Source: CAD feature listing. Evaluate the final solid. Frame: model axes, mm. Round coordinates to 2 decimals unless told otherwise and drop trailing zeros. Order: outer loops, then holes, each group sorted by start corner. A loop starts at its lowest first (then second) coordinate and runs counter-clockwise, first axis right, second up. Notation, with made-up numbers: (79.5, 41.25) - (130.5, 41.25) arc R16 ccw to (130.5, 52.25) - close; hole circle Ø7 at (-4, 75.5). An arc over 180 degrees is marked (long way). Return JSON: item names as keys, results as strings. Group by question number.
1) Ray query, line 1 (X direction, y = 1.75, z = -31.75) (3 decimals); line 2 (X direction, y = 0.9, z = -12.7); line 3 (X direction, y = 0.75, z = -30) (3 decimals). Return the intervals inside material, ascending. Write a range as from..to.
2) Section D-D, the plane x = -38.1. Return loops of the section in (y, z).
3) Contact query for a flat-ended pin moving along its axis: P1, Ø4, axis at x = -55.5, z = -68, coming from the -Y side. Output: stop coordinate, or through.
4) Section B-B, the plane z = -57.15. Return loops of the section in (x, y).
5) Section A-A, the plane z = -36.5. Return loops of the section in (x, y) (3 decimals), plus the area to 3 significant figures.
6) Section C-C, the plane x = -63.5. Return loops of the section in (y, z), plus the area to 3 significant figures.
Autodesk Inventor part; units mm, degrees
ref_plane "YZ Plane" through (0, 0, 0) normal (1, 0, 0) x (0, 1, 0)
ref_plane "XZ Plane" through (0, 0, 0) normal (0, 1, 0) x (-1, 0, 0)
ref_plane "XY Plane" through (0, 0, 0) normal (0, 0, 1) x (1, 0, 0)
sketch "Sketch1" plane through (0, 0, 0) normal (0, 1, 0) x (-1, 0, 0)
  line L0 (0, 0) -> (76.2, 0)
  line L1 (76.2, 0) -> (76.2, -76.2)
  line L2 (76.2, -76.2) -> (0, -76.2)
  line L3 (0, -76.2) -> (0, 0)
  dimension "d0" = 76.2
  dimension "d1" = 76.2
extrude "Extrusion1" add sketch "Sketch1" along normal blind 2.3813
sketch "Sketch2" plane through (0, 2.3813, 0) normal (0, 1, 0) x (1, 0, 0)
  line L0 (-83.8553, 12.7) -> (21.3104, 12.7) construction
  line L1 (-76.2, 0) -> (0, 0) construction
  line L2 (-76.2, 76.2) -> (-76.2, 0) construction
  point P0 (-63.5, 12.7)
  point P1 (-38.1, 12.7)
  point P2 (-12.7, 12.7)
  dimension "d4" = 12.7
  dimension "d5" = 12.7
  dimension "d6" = 25.4
  dimension "d39" = 25.4
hole "Hole1" at (-63.5, 2.3813, -12.7) at (-38.1, 2.3813, -12.7) at (-12.7, 2.3813, -12.7) direction (0, -1, 0) diameter 4.4958 end through all
sketch "Sketch3" plane through (0, 2.3813, 0) normal (0, 1, 0) x (1, 0, 0)
  line L0 (-85.7811, 31.75) -> (14.4142, 31.75) construction
  line L1 (-76.2, 0) -> (0, 0) construction
  line L2 (-38.1, 80.8292) -> (-38.1, -11.6218) construction
  line L3 (0, 76.2) -> (-76.2, 76.2) construction
  point P0 (-58.3565, 31.75)
  point P1 (-17.8435, 31.75)
  point P2 (-38.1, 76.2)
  dimension "d14" = 31.75
  dimension "d16" = 40.513
hole "Hole2" at (-58.3565, 2.3813, -31.75) at (-17.8435, 2.3813, -31.75) direction (0, -1, 0) diameter 3.175 end through all
sketch "Sketch4" plane through (0, 2.3813, 0) normal (0, 1, 0) x (1, 0, 0)
  line L0 (-58.3565, 76.2) -> (-17.8435, 76.2)
  line L1 (-17.8435, 76.2) -> (-17.8435, 38.1)
  line L2 (-17.8435, 38.1) -> (-58.3565, 38.1)
  line L3 (-58.3565, 38.1) -> (-58.3565, 76.2)
  line L4 (0, 76.2) -> (-76.2, 76.2)
  line L5 (-38.1, 81.963) -> (-38.1, -24.4331)
  line L6 (-76.2, 0) -> (0, 0)
  line L7 (-53.975, 38.1) -> (-22.225, 38.1)
  line L8 (-22.225, 38.1) -> (-22.225, 25.4)
  line L9 (-22.225, 25.4) -> (-53.975, 25.4)
  line L10 (-53.975, 25.4) -> (-53.975, 38.1)
  point P0 (-38.1, 0)
  dimension "d24" = 38.1
  dimension "d27" = 31.75
  dimension "d28" = 12.7
  dimension "d29" = 40.513
extrude "Extrusion2" cut sketch "Sketch4" against normal blind 2.3813
sketch "Sketch5" plane through (0, 2.3813, 0) normal (0, 1, 0) x (1, 0, 0)
  line L0 (-81.1122, 57.15) -> (21.0892, 57.15) construction
  line L1 (-58.3565, 76.2) -> (-76.2, 76.2) construction
  line L2 (-38.1, 88.2697) -> (-38.1, -12.0157) construction
  line L3 (-76.2, 0) -> (0, 0) construction
  point P0 (-64.897, 57.15)
  point P1 (-11.303, 57.15)
  point P2 (-38.1, 0)
  dimension "d30" = 19.05
  dimension "d31" = 53.594
hole "Hole3" at (-64.897, 2.3813, -57.15) at (-11.303, 2.3813, -57.15) direction (0, -1, 0) diameter 6.35 end through all
properties part number "dmc_plate"
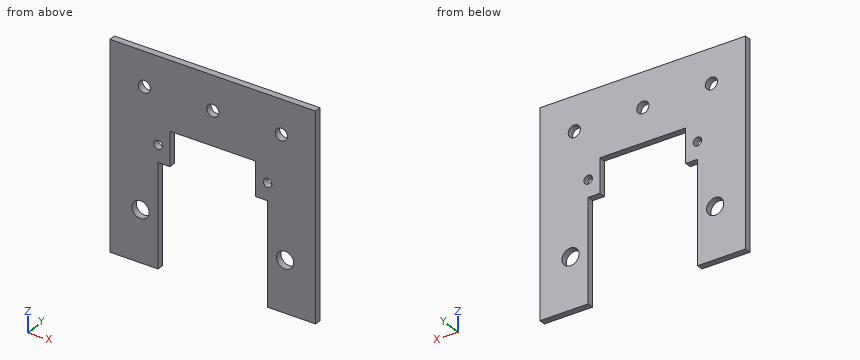
Geometry check:
{
 "1": {"line 1": "-76.2..-59.944, -56.769..-53.975, -22.225..-19.431, -16.256..0", "line 2": "-76.2..-65.75, -61.25..-40.35, -35.85..-14.95, -10.45..0", "line 3": "-76.2..-53.975, -22.225..0"},
 "2": {"outline": "(0, -25.4) - (2.38, -25.4) - (2.38, -14.95) - (0, -14.95) - close; (0, -10.45) - (2.38, -10.45) - (2.38, 0) - (0, 0) - close"},
 "3": {"P1": "through"},
 "4": {"outline": "(-76.2, 0) - (-68.07, 0) - (-68.07, 2.38) - (-76.2, 2.38) - close; (-61.72, 0) - (-58.36, 0) - (-58.36, 2.38) - (-61.72, 2.38) - close; (-17.84, 0) - (-14.48, 0) - (-14.48, 2.38) - (-17.84, 2.38) - close; (-8.13, 0) - (0, 0) - (0, 2.38) - (-8.13, 2.38) - close"},
 "5": {"outline": "(-76.2, 0) - (-53.975, 0) - (-53.975, 2.381) - (-76.2, 2.381) - close; (-22.225, 0) - (0, 0) - (0, 2.381) - (-22.225, 2.381) - close", "area": "106 mm2"},
 "6": {"outline": "(0, -76.2) - (2.38, -76.2) - (2.38, -60) - (0, -60) - close; (0, -54.3) - (2.38, -54.3) - (2.38, -14.95) - (0, -14.95) - close; (0, -10.45) - (2.38, -10.45) - (2.38, 0) - (0, 0) - close", "area": "157 mm2"}
}
